Could you check a few things on this model? Use its own coordinates, in mm. A direction names the side the tool comes from. Give positions to 0.01 mm unless a question says otherwise; leave off trailing zeros. Order: outer loops, then holes, each group sorted by start corner. A loop starts at its lowest first (then second) coordinate and runs counter-clockwise, first axis right, second up. Notation, with made-up numbers: (12.5, 7) - (46.5, 7) arc R22 cw to (46.5, 43) - close; hole circle Ø4 at (-6.75, 52.5). An arc over 180 degrees is marked (long way). Put each result on its own line as item: value.
from build123d import *

# Parameters (mm, degrees)
SKETCH1_R           = 10
BOSS_EXTRUDE1_DEPTH = 15
SKETCH2_R           = 10
CUT_EXTRUDE1_DEPTH  = 57.124860802
FILLET1_R           = 15


with BuildPart() as part:
    # Sketch1 → Boss-Extrude1 (new, symmetric)
    with BuildSketch(Plane(origin=(0, 0, 0), x_dir=(1, 0, 0), z_dir=(0, 1, 0))):
        Polygon((-45, 15), (15, 15), (15, -15), (-45, -15), (-45, -5), (-15, -5), (-15, 5), (-45, 5), align=None)
        with Locations(Location((0, 0, 0), (0, 0, 270))):
            Circle(SKETCH1_R, mode=Mode.SUBTRACT)
    extrude(amount=BOSS_EXTRUDE1_DEPTH, both=True)

    # Sketch2 → Cut-Extrude1 (cut, through all)
    with BuildSketch(Plane.XY.offset(15)):
        with Locations((-30, 0)):
            Circle(SKETCH2_R)
    extrude(amount=-CUT_EXTRUDE1_DEPTH, mode=Mode.SUBTRACT)

    # Fillet1
    fillet1_edges = [part.edges().sort_by_distance(p)[0] for p in [
        (-45, -15, -10),
        (-45, 15, -10),
        (-45, -15, 10),
        (-45, 15, 10),
    ]]
    fillet(fillet1_edges, radius=FILLET1_R - 0.0001)  # a hair under: the kernel refuses the full size


solid = part.part
1) If I drill on line 1 (X direction, y = -0.5, z = 8.5); line 2 (X direction, y = 5.5, z = -8.25); line 3 (Y direction, x = -30, z = 11), over which ranges is the centre line in solid material (lowest first)? Write a range as [from, to].
Filled in:
line 1: x = [-44.99, -39.99], [-20.01, -5.27], [5.27, 15]
line 2: x = [-43.96, -38.35], [-21.65, -5.65], [5.65, 15]
line 3: y = [-15, -10], [10, 15]
2) We'd pull the mould along Y, two halves only. Please class faces 1 (the flat face through (-9, 0, -15)), 2 (the cylindrical face through (-40.49, -10.72, 9.93)), 3 (the cylindrical face through (-40, 0, 10)): pulls with the +Y half, pulls with the -Y half, needs draft (parallel to the pull), parting line crosses it, or undercut.
Filled in:
face 1: needs draft
face 2: pulls with the -Y half
face 3: undercut
3) Suppose I cut it at D-D, the plane y = -2.5. List the corners of the cut face in (x, z) for me.
Filled in:
outline: (-44.79, -15) - (-39.68, -15) - (-39.68, -5) - (-44.79, -5) - close; (-44.79, 5) - (-39.68, 5) - (-39.68, 15) - (-44.79, 15) - close; (-20.32, -15) - (15, -15) - (15, 15) - (-20.32, 15) - (-20.32, 5) - (-15, 5) - (-15, -5) - (-20.32, -5) - close; hole circle Ø20 at (0, 0)
4) Suppose I cut it at A-A, the plane z = 7. State how many separate pieces and enclosed holes the cut face has, and give its area (3 significant figures).
Filled in:
separate pieces: 2
enclosed holes: 1
area: 961 mm^2
5) Which directions (+Z, -Z, +X, -X, +Y, -Y) give clear straight access to the entire face, cutting with the end or side of a thin tool? Please do faces 4 (the flat face through (-19.8, 0.2, -5)), 5 (the cylindrical face through (-40.49, 10.72, 9.93)).
Filled in:
face 4: -X, +Y, -Y
face 5: +Z, -Z, -X, +Y
6) I'm going to push flat-ended pins straight in: pin 1 (16 mm diameter, centred on x = -30, y = 0, fed in from +Z); pin 2 (1.5 mm diameter, centred on y = 3.5, z = 9, fed in from -X); pin 3 (5 mm diameter, centred on y = -7, z = 1.5, fed in from -X). Where does each tip first touch, or does it pass through?
Filled in:
pin 1: passes through
pin 2: stops at x = -44.75
pin 3: stops at x = -15
7) Suppose I cut it at B-B, the plane x = 0. List the corners of the cut face in (y, z) for me.
Filled in:
outline: (-15, -15) - (15, -15) - (15, -10) - (-15, -10) - close; (-15, 10) - (15, 10) - (15, 15) - (-15, 15) - close
